Verification items for the finished model (mm, model axes). A direction names the side the tool comes from. Give positions to 0.01 mm unless a question says otherwise; leave off trailing zeros. Order: outer loops, then holes, each group sorted by start corner. A loop starts at its lowest first (then second) coordinate and runs counter-clockwise, first axis right, second up.
from build123d import *

# Parameters (mm, degrees)
F1_DEPTH = 4.5


with BuildPart() as f1:
    # F0 (on Top) → F1 (new body, symmetric)
    with BuildSketch(Plane.XY):
        with BuildLine():
            Line((-27, -3), (-27, 0))
            Line((-27, 0), (-12.5, 0))
            Line((-12.5, 0), (-12.5, 7))
            ThreePointArc((-12.5, 7), (-11.6213203436, 9.1213203436), (-9.5, 10))
            Line((-9.5, 10), (9.5, 10))
            ThreePointArc((9.5, 10), (11.6213203436, 9.1213203436), (12.5, 7))
            Line((12.5, 7), (12.5, 0))
            Line((12.5, 0), (27, 0))
            Line((27, 0), (27, -3))
            Line((27, -3), (35, -18))
            Line((35, -18), (37, -18))
            Line((37, -18), (37, 0))
            Line((37, 0), (32.1797316785, 104.8762590077))
            Line((32.1797316785, 104.8762590077), (27.1827775434, 105.0507564913))
            Line((27.1827775434, 105.0507564913), (27.0780790533, 102.0525840102))
            Line((27.0780790533, 102.0525840102), (22.0811249182, 102.2270814937))
            Line((22.0811249182, 102.2270814937), (19.2220026408, 20.3525317921))
            ThreePointArc((19.2220026408, 20.3525317921), (18.2698252399, 18.2631691773), (16.1191316696, 17.4590578011))
            Line((16.1191316696, 17.4590578011), (-14.8619839679, 18.5409421989))
            ThreePointArc((-14.8619839679, 18.5409421989), (-16.9513465827, 19.4931195998), (-17.7554579589, 21.6438131701))
            Line((-17.7554579589, 21.6438131701), (-14.8963356815, 103.5183628717))
            Line((-14.8963356815, 103.5183628717), (-19.8932898166, 103.6928603552))
            Line((-19.8932898166, 103.6928603552), (-19.7885913265, 106.6910328363))
            Line((-19.7885913265, 106.6910328363), (-24.7855454616, 106.8655303198))
            Line((-24.7855454616, 106.8655303198), (-37, 0))
            Line((-37, 0), (-37, -18))
            Line((-37, -18), (-35, -18))
            Line((-35, -18), (-27, -3))
        make_face()
    extrude(amount=F1_DEPTH, both=True)


solid = f1.part
(1) Go/stop test with flat-tipped pins: pin 1 (1 mm diameter, centred on y = 61, z = -3, fed in from +X); pin 2 (1.5 mm diameter, centred on y = 76.5, z = -2, fed in from -X); pin 3 (4 mm diameter, centred on y = 43.5, z = 2.5, fed in from -X). Record where each tip stops, or that it passes through.
Solved:
pin 1: stops at x = 34.22
pin 2: stops at x = -28.34
pin 3: stops at x = -32.26
(2) Section check A-A, the plane y = -6.5. Enter the section's corners in (x, z), then the cut area to 3 significant figures.
Solved:
outline: (-37, -4.5) - (-28.87, -4.5) - (-28.87, 4.5) - (-37, 4.5) - close; (28.87, -4.5) - (37, -4.5) - (37, 4.5) - (28.87, 4.5) - close
area: 146 mm2
(3) Release check for a two-part mould opening along Y. For faces 3 (the flat face through (30.944, -10.395, 0.063)), 4 (the flat face through (-12.5, 3, 0)), 5 (the cylindrical face through (-16.93, 19.47, 0.06)) record: pulls with the +Y half, pulls with the -Y half, needs draft (parallel to the pull), parting line crosses it, or undercut.
Solved:
face 3: pulls with the -Y half
face 4: needs draft
face 5: undercut
(4) Set-up check for faces 1 (the flat face through (-27, -2, 0)), 2 (the flat face through (24, 45, -4.5)): record each of +Z, -Z, +X, -X, +Y, -Y from which the full face is reachable in a straight line by a thin tool's end or side.
Solved:
face 1: +Z, -Z, -Y
face 2: -Z, +X, -X, +Y, -Y
(5) Section check D-D, the plane x = 8. Enter the section's corners in (y, z).
Solved:
outline: (10, -4.5) - (17.74, -4.5) - (17.74, 4.5) - (10, 4.5) - close
(6) Section check C-C, the plane y = 64. Enter the section's corners in (x, z).
Solved:
outline: (-29.68, -4.5) - (-16.28, -4.5) - (-16.28, 4.5) - (-29.68, 4.5) - close; (20.75, -4.5) - (34.06, -4.5) - (34.06, 4.5) - (20.75, 4.5) - close
(7) Scan lines: line 1 (X direction, y = -0.5, z = 1.5); line 2 (X direction, y = 84.5, z = 3.25); line 3 (Y direction, x = 12, z = 2.25). Record each from-to range of solid material in increasing order.
Solved:
line 1: x = -37 to -27, 27 to 37
line 2: x = -27.34 to -15.56, 21.46 to 33.12
line 3: y = 8.66 to 17.6
(8) Section check B-B, the plane z = 3.25. Enter the section's corners in (x, y).
Solved:
outline: (-37, -18) - (-35, -18) - (-27, -3) - (-27, 0) - (-12.5, 0) - (-12.5, 7) arc R3 cw to (-9.5, 10) - (9.5, 10) arc R3 cw to (12.5, 7) - (12.5, 0) - (27, 0) - (27, -3) - (35, -18) - (37, -18) - (37, 0) - (32.18, 104.88) - (27.18, 105.05) - (27.08, 102.05) - (22.08, 102.23) - (19.22, 20.35) arc R3 cw to (16.12, 17.46) - (-14.86, 18.54) arc R3 cw to (-17.76, 21.64) - (-14.9, 103.52) - (-19.89, 103.69) - (-19.79, 106.69) - (-24.79, 106.87) - (-37, 0) - close
